```python
from build123d import *

# Parameters (mm, degrees)
F1_DEPTH = 685.8
F2_R     = 76.2


with BuildPart() as f1:
    # F0 (on Front) → F1 (new body)
    with BuildSketch(Plane.XZ):
        with BuildLine():
            ThreePointArc((-1168.4, 0), (0, 437.803955), (1168.4, 0))
            Line((1168.4, 0), (1168.4, 1320.8))
            ThreePointArc((1168.4, 1320.8), (0, 1758.603955), (-1168.4, 1320.8))
            Line((-1168.4, 1320.8), (-1168.4, 0))
        make_face()
    extrude(amount=F1_DEPTH)

    # F2
    f2_edges = [f1.edges().sort_by_distance(p)[0] for p in [
        (0, -685.8, 1758.603955),
        (-1168.4, -685.8, 660.4),
        (0, -685.8, 437.803955),
        (1168.4, -685.8, 660.4),
        (1168.4, -342.9, 1320.8),
        (-1168.4, -342.9, 1320.8),
        (0, 0, 1758.603955),
        (1168.4, -342.9, 0),
        (1168.4, 0, 660.4),
        (-1168.4, -342.9, 0),
        (-1168.4, 0, 660.4),
    ]]
    fillet(f2_edges, radius=F2_R)


solid = f1.part
```
Model file for the job. Use its own axes, mm. Give positions to 0.01 mm unless a question says otherwise; leave off trailing zeros. Loops run counter-clockwise (first coordinate to the right, second up) from the corner with the lowest first, then second, coordinate; pieces in that order, holes last. Notation, with made-up numbers: (27, -40) - (67, -40) arc R14 cw to (67, -15) - close; hole circle Ø6 at (25, -3.75). An arc over 180 degrees is marked (long way). One line per item, written item: value. Start each with the question number.
1. Pin check, flat tips, straight feed: pin 1 (4 mm diameter, centred on x = 311.5, z = 435.5, fed in from -Y); pin 2 (10 mm diameter, centred on x = -437, y = -343.5, fed in from -Z). Stop position of each tip, or through.
2. Slice it at A-A (y = -432.5). List the corners of the cut face in (x, z), plus the area to 3 significant figures.
3. Pull direction X, two halves, no side cores. Call faces 1 (the cylindrical face through (1125.691, -309.067, 89.743)), 2 (the flat face through (1168.4, -339, 714)), 3 (the cylindrical face through (-15.679, -300.533, 437.735)), 4 (the cylindrical face through (17.35, -339.17, 1758.52)): pulls with the +X half, pulls with the -X half, needs draft (parallel to the pull), parting line crosses it, or undercut.
4. Probe L1, parallel to X at y = -567.5, z = 290.5; L2, parallel to Z at x = 39, y = -172.5; L3, parallel to Z at x = -186.5, y = -413. List the from-to ranges inside material, lowest first. Write a range as from..to.
Solution:
1. pin 1: stops at y = -667.63
1. pin 2: stops at z = 381.99
2. outline: (-1168.4, 158.19) arc R76.2 ccw to (-1047.32, 96.61) arc R1778 cw to (1047.32, 96.61) arc R76.2 ccw to (1168.4, 158.19) - (1168.4, 1285.68) arc R76.2 ccw to (1141.1, 1344.12) arc R1778 ccw to (-1141.1, 1344.12) arc R76.2 ccw to (-1168.4, 1285.68) - close
2. area: 3,080,000 mm^2
3. face 1: undercut
3. face 2: pulls with the +X half
3. face 3: undercut
3. face 4: parting line crosses it
4. L1: x = -1168.4..-708.6, 708.6..1168.4
4. L2: z = 437.38..1758.18
4. L3: z = 428..1748.8
